```python
from build123d import *

# Parameters (mm, degrees)
SKETCH_1_R          = 29.5
EXTRUDE_1_DEPTH     = 5
SKETCH_2_W          = 28.166253132
SKETCH_2_H          = 32.95394871
CUT_EXTRUDE_1_DEPTH = 43.017853348
SKETCH_6_R          = 1.6
CUT_EXTRUDE_5_DEPTH = 40.587441773


with BuildPart() as part:
    # 草图1 → 凸台-拉伸1 (new body)
    with BuildSketch(Plane(origin=(0, 0, 0), x_dir=(1, 0, 0), z_dir=(0, 1, 0))):
        with Locations(Location((0, 0, 0), (0, 0, 270))):
            Circle(SKETCH_1_R)
    extrude(amount=EXTRUDE_1_DEPTH)

    # 草图2 → 切除-拉伸1 (cut, through all)
    with BuildSketch(Plane(origin=(0, 5, 0), x_dir=(1, 0, 0), z_dir=(0, 1, 0))):
        with Locations((0, 29.5)):
            Rectangle(SKETCH_2_W, SKETCH_2_H)
        with Locations((0, -29.5)):
            Rectangle(SKETCH_2_W, SKETCH_2_H)
    extrude(amount=-CUT_EXTRUDE_1_DEPTH, mode=Mode.SUBTRACT)

    # 草图6 → 切除-拉伸5 (cut, through all)
    with BuildSketch(Plane(origin=(0, 5, 0), x_dir=(1, 0, 0), z_dir=(0, 1, 0))):
        with Locations(Location((-21.376, 12.613, 0), (0, 0, 270))):
            Circle(SKETCH_6_R)
        with Locations(Location((-21.376, -12.613, 0), (0, 0, 270))):
            Circle(SKETCH_6_R)
        with Locations(Location((21.376, 12.613, 0), (0, 0, 270))):
            Circle(SKETCH_6_R)
        with Locations(Location((21.376, -12.613, 0), (0, 0, 270))):
            Circle(SKETCH_6_R)
    extrude(amount=-CUT_EXTRUDE_5_DEPTH, mode=Mode.SUBTRACT)


solid = part.part
```
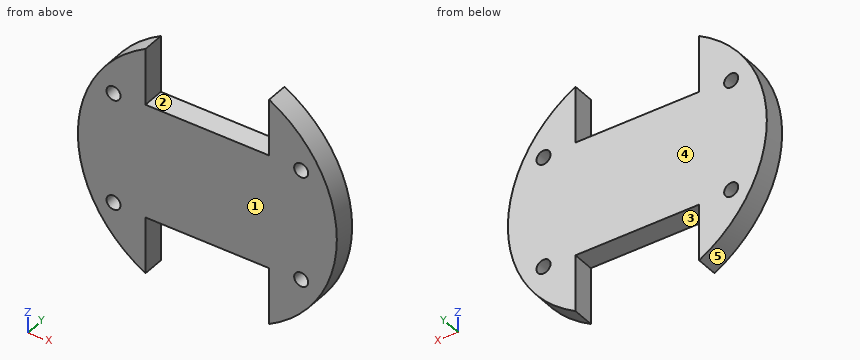
Geometry check sheet. Reference: the model listing, model coordinates, mm. Face numbers are marked on the shaded views. A direction names the side the tool comes from. Coordinates: 2 decimals unless noted, no trailing zeros. Write each loop counter-clockwise with the first axis right and the second up, starting at its lowest first coordinate (ties: lowest second). Pieces come first, ordered by that corner, then holes. Notation, with made-up numbers: (-18.5, 2.25) -> (22.5, 2.25) arc R29 cw to (22.5, 38.25) -> close; hole circle Ø8 at (66, 27). An arc over 180 degrees is marked (long way). Use CSV: the item, a comma, the result in double quotes. Start each with the question number.
Item 1: Cross-section at A-A, the plane z = -12. Record the cut outline in (x, y), plus the area to 3 significant figures.
Item 2: Cross-section at B-B, the plane y = 2.25. Record the cut outline in (x, z).
Item 3: Set-up check for the marked faces 1 and 2: record each of +Z, -Z, +X, -X, +Y, -Y from which the full face is reachable in a straight line by a thin tool's end or side.
Item 4: Cross-section at C-C, the plane z = 21. Record the cut outline in (x, y).
Item 5: Thickness scan on line 1 (Z direction, x = 21, y = 4.7); line 2 (X direction, y = 3, z = -22); line 3 (X direction, y = 2, z = 20.5). Record the ranges inside material, lowest first.
Item 6: Cross-section at D-D, the plane x = 7. Record the cut outline in (y, z), plus the area to 3 significant figures.
Item 7: Depth check by flat-ended pin: pin 1 Ø1.5 at (x, y) = (4.5, 1.5) entering from +Z; pin 2 Ø3 at (x, z) = (-14, 18) entering from +Y; pin 3 Ø1.5 at (x, y) = (-7, 1.5) entering from -Z; pin 4 Ø1.5 at (y, z) = (1, -15) entering from -X. Enter the tip coordinate at first touch or a pass-through.
Item 8: Mould release check, pull along X, two halves, no side actions. Record for the marked faces 3, 4 and 5: released by +X, released by -X, zero draft, split by the parting line, or undercut.
Answers:
1,outline,"(-26.95, 0) -> (-22.85, 0) -> (-22.85, 5) -> (-26.95, 5) -> close; (-19.9, 0) -> (19.9, 0) -> (19.9, 5) -> (-19.9, 5) -> close; (22.85, 0) -> (26.95, 0) -> (26.95, 5) -> (22.85, 5) -> close"
1,area,"240 mm^2"
2,outline,"(-14.08, -25.92) -> (-14.08, -13.02) -> (14.08, -13.02) -> (14.08, -25.92) arc R29.5 ccw to (14.08, 25.92) -> (14.08, 13.02) -> (-14.08, 13.02) -> (-14.08, 25.92) arc R29.5 ccw to start; hole circle Ø3.2 at (-21.38, -12.61); hole circle Ø3.2 at (-21.38, 12.61); hole circle Ø3.2 at (21.38, -12.61); hole circle Ø3.2 at (21.38, 12.61)"
3,face 1,"+Z, -Z, +X, -X, -Y"
3,face 2,"+Z, +Y, -Y"
4,outline,"(-20.72, 0) -> (-14.08, 0) -> (-14.08, 5) -> (-20.72, 5) -> close; (14.08, 0) -> (20.72, 0) -> (20.72, 5) -> (14.08, 5) -> close"
5,line 1,"-20.72 to -14.17, -11.06 to 11.06, 14.17 to 20.72"
5,line 2,"-19.65 to -14.08, 14.08 to 19.65"
5,line 3,"-21.21 to -14.08, 14.08 to 21.21"
6,outline,"(0, -13.02) -> (5, -13.02) -> (5, 13.02) -> (0, 13.02) -> close"
6,area,"130 mm^2"
7,pin 1,"z = 13.02"
7,pin 2,"y = 5"
7,pin 3,"z = -13.02"
7,pin 4,"x = -25.83"
8,face 3,"undercut"
8,face 4,"zero draft"
8,face 5,"released by -X"
